```python
from build123d import *

# Parameters (mm, degrees)
F0_W     = 73.025
F0_H     = 38.1
F1_DEPTH = 3.175
F2_W     = 73.025
F2_H     = 34.925
F3_DEPTH = 3.175
F5_D     = 3.2
F5_DEPTH = 34.925
F5_TIP   = 0.9613769904
F7_DEPTH = 3.176
F8_W     = 34.925
F8_H     = 34.925
F9_DEPTH = 3.176
F10_R    = 3.17499
F11_R    = 4.7625


# Not quite as in the source:
# - a fillet or chamfer is up to 0.001 mm smaller than in the source, because OpenCascade refuses the exact size


with BuildPart() as f1:
    # F0 (on Front) → F1 (new body)
    with BuildSketch(Plane.XZ):
        Rectangle(F0_W, F0_H)
    extrude(amount=F1_DEPTH)

    # F2 (on face) → F3 (join)
    with BuildSketch(Plane.XY.offset(19.05)):
        with Locations((0, -20.6375)):
            Rectangle(F2_W, F2_H)
    extrude(amount=-F3_DEPTH)

    # F5
    with Locations(Plane.XZ.offset(3.175)):
        with Locations((-27.78125, -4.05)):
            Hole(F5_D / 2, depth=F5_DEPTH)
            with Locations((0, 0, -(F5_DEPTH + F5_TIP / 2))):  # 118° drill point
                Cone(0, F5_D / 2, F5_TIP, mode=Mode.SUBTRACT)

    # F6 (on face) → F7 (cut, through all)
    with BuildSketch(Plane(origin=(0, 0, 15.875), x_dir=(1, 0, 0), z_dir=(0, 0, -1))):
        with BuildLine():
            ThreePointArc((5.13125, 7.9375), (7.5125, 5.55625), (9.89375, 7.9375))
            Line((9.89375, 7.9375), (9.89375, 26.9875))
            ThreePointArc((9.89375, 26.9875), (7.5125, 29.36875), (5.13125, 26.9875))
            Line((5.13125, 26.9875), (5.13125, 7.9375))
        make_face()
        with BuildLine():
            ThreePointArc((23.13125, 7.9375), (25.5125, 5.55625), (27.89375, 7.9375))
            Line((27.89375, 7.9375), (27.89375, 26.9875))
            ThreePointArc((27.89375, 26.9875), (25.5125, 29.36875), (23.13125, 26.9875))
            Line((23.13125, 26.9875), (23.13125, 7.9375))
        make_face()
    extrude(amount=-F7_DEPTH, mode=Mode.SUBTRACT)

    # F8 (on face) → F9 (cut, through all)
    with BuildSketch(Plane.XZ.offset(3.175)):
        with Locations((19.05, -1.5875)):
            Rectangle(F8_W, F8_H)
    extrude(amount=-F9_DEPTH, mode=Mode.SUBTRACT)

    # F10 (radius 3.175 in the source; OpenCascade refuses exactly that, so slightly less here)
    f10_edges = [f1.edges().sort_by_distance(p)[0] for p in [
        (0, -38.1, 15.875),
        (-17.4625, -3.175, -19.05),
    ]]
    fillet(f10_edges, radius=F10_R)

    # F11
    f11_edges = [f1.edges().sort_by_distance(p)[0] for p in [
        (1.5875, -1.5875, 15.875),
    ]]
    fillet(f11_edges, radius=F11_R)


solid = f1.part
```
Could you check a few things on this model? Use its own coordinates, in mm. A direction names the side the tool comes from. Round coordinates to 2 decimals unless told otherwise and drop trailing zeros. Loops run counter-clockwise (first coordinate to the right, second up) from the corner with the lowest first, then second, coordinate; pieces in that order, holes last. Notation, with made-up numbers: M 57,-22 L 109,-22 A14 cw 109,-3 Z; hole C 39.5,1 d6. An arc over 180 degrees is marked long. Put each result on its own line as item: value.
Q1. Thinking about a two-plate mould opening in X: for faces 4 (the face through (25.56, -29.37, 17.44)), 5 (the face through (-17, 0, 0)), 6 (the face through (1.588, -2, -4)), 7 (the face through (9.894, -17, 17)), which applies, released by +X, released by -X, zero draft, split by the parting line, or undercut?
Check result:
face 4: undercut
face 5: zero draft
face 6: released by +X
face 7: undercut
Q2. I need wall thicknesses on probe 1 along X at (y, z) = (-1, -4); probe 2 along Z at (x, y) = (-22, -13) (3 decimals); probe 3 along Y at (x, z) = (0.5, -15.5) (3 decimals). Which ranges of each line are inside material? Lowest first, please.
Check result:
probe 1: -36.51 to -29.38, -26.18 to 1.59
probe 2: 15.875 to 19.05
probe 3: -3.175 to 0
Q3. Imagine slicing it at B-B (z = -4.05). Write out the boundary of the cut face in (x, y) (1 decimal), then the cut area to 3 significant figures.
Check result:
outline: M -36.5,-3.2 L -29.4,-3.2 L -29.4,0 L -36.5,0 Z; M -26.2,-3.2 L 1.6,-3.2 L 1.6,0 L -26.2,0 Z
area: 111 mm2
Q4. On a 3-axis mill with a long thin cutter (end or side, diameter ignored), from which of +Z, -Z, +X, -X, +Y, -Y can I reach the whole of each face in a straight line? I mean faces 1 (the face through (-20, -3.175, 0)), 2 (the face through (3, -1.6, 14.5)), 3 (the face through (23.131, -18, 17)). Say none if no direction works.
Check result:
face 1: -Z, +X, -X, -Y
face 2: -Z, +X, +Y, -Y
face 3: +Z, -Z
Q5. For pin 1 (4 mm diameter, centred on x = 27.5, y = -31.5, fed in from -Z) (3 decimals); pin 2 (1.9 mm diameter, centred on x = -27.78, z = -4.05, fed in from +Y); pin 3 (3.5 mm diameter, centred on y = -1.5, z = -8.5, fed in from +X); pin 4 (6 mm diameter, centred on x = 7, y = -21, fed in from +Z), each with a flat end and sliding along its axis, tell me the tip position at first contact or that it passes through.
Check result:
pin 1: z = 15.875
pin 2: through
pin 3: x = 1.59
pin 4: z = 19.05
Q6. Imagine slicing it at A-A (y = -25). State how many separate pieces and enclosed holes the cut face has, then the cut area to 3 significant figures.
Check result:
separate pieces: 3
enclosed holes: 0
area: 202 mm2
